Input: part model. Units: mm. Frame: model coordinates. A direction names the side the tool comes from. Give positions to 0.01 mm unless a question says otherwise; leave off trailing zeros. Loops run counter-clockwise (first coordinate to the right, second up) from the corner with the lowest first, then second, coordinate; pieces in that order, holes last.
from build123d import *

# Parameters (mm, degrees)
F0_R          = 25.4
F1_DEPTH      = 19.05
F2_R          = 6.35
F3_DEPTH      = 12.7
F5_DEPTH      = 25.4
F5_DEPTH_BACK = 50.8
F6_W          = 25.4
F6_H          = 25.4
F7_DEPTH      = 25.4
F9_DEPTH      = 115.8426897829


# Not quite as in the source:
# - a pattern or mirror of a feature is missing from the dataset's text; its kind, count and spacing are read off the source's solid


with BuildPart() as f1:
    # F0 (on Top) → F1 (new body)
    with BuildSketch(Plane.XY):
        with BuildLine():
            Line((-35.052, -28.575), (35.052, -28.575))
            Line((35.052, -28.575), (35.052, 28.575))
            ThreePointArc((35.052, 28.575), (28.9292508026, 48.3674518946), (12.7, 61.2453643077))
            Line((12.7, 61.2453643077), (12.7, 79.375))
            Line((12.7, 79.375), (-12.7, 79.375))
            Line((-12.7, 79.375), (-12.7, 61.2453643077))
            ThreePointArc((-12.7, 61.2453643077), (-28.9292508026, 48.3674518946), (-35.052, 28.575))
            Line((-35.052, 28.575), (-35.052, -28.575))
        make_face()
        with Locations((0, 28.575)):
            Circle(F0_R, mode=Mode.SUBTRACT)
    extrude(amount=F1_DEPTH)

    # F2 (on face) → F3 (join)
    with BuildSketch(Plane(origin=(-35.052, 0, 0), x_dir=(0, -1, 0), z_dir=(-1, 0, 0))):
        with BuildLine():
            Line((3.175, 19.05), (28.575, 19.05))
            Line((28.575, 19.05), (28.575, 44.45))
            ThreePointArc((28.575, 44.45), (15.875, 57.15), (3.175, 44.45))
            Line((3.175, 44.45), (3.175, 19.05))
        make_face()
        with Locations((15.875, 44.45)):
            Circle(F2_R, mode=Mode.SUBTRACT)
    f3 = extrude(amount=-F3_DEPTH)

    # F3_copies: F3 across plane
    add(f3.mirror(Plane(origin=(0, 0, 0), x_dir=(0, 0, 1), z_dir=(1, 0, 0))))

    # F4 (on face) → F5 (join, two sides)
    with BuildSketch(Plane(origin=(-12.7, 0, 0), x_dir=(0, -1, 0), z_dir=(-1, 0, 0))) as f5_sk:
        Polygon((-79.375, 0), (-79.375, 19.05), (-178.3617036526, -38.1), (-170.1128116815, -52.3875), align=None)
    extrude(amount=F5_DEPTH)
    extrude(f5_sk.sketch, amount=-F5_DEPTH_BACK)

    # F6 (on face) → F7 (cut)
    with BuildSketch(Plane(origin=(0, 28.092641971, 48.6578832127), x_dir=(1, 0, 0), z_dir=(0, 0.5, 0.8660254038))):
        with Locations((25.4, 71.9157664254)):
            Rectangle(F6_W, F6_H)
        with Locations((-25.4, 71.9157664254)):
            Rectangle(F6_W, F6_H)
        with BuildLine():
            ThreePointArc((-38.1, 135.4157664254), (-26.9407683632, 162.3565347886), (0, 173.5157664254))
            Line((0, 173.5157664254), (-38.1, 173.5157664254))
            Line((-38.1, 173.5157664254), (-38.1, 135.4157664254))
        make_face()
        with BuildLine():
            ThreePointArc((0, 173.5157664254), (26.9407683632, 162.3565347886), (38.1, 135.4157664254))
            Line((38.1, 135.4157664254), (38.1, 173.5157664254))
            Line((38.1, 173.5157664254), (0, 173.5157664254))
        make_face()
    extrude(amount=-F7_DEPTH, mode=Mode.SUBTRACT)

    # F8 (on face) → F9 (cut, through all)
    with BuildSketch(Plane(origin=(0, 28.092641971, 48.6578832127), x_dir=(1, 0, 0), z_dir=(0, 0.5, 0.8660254038))):
        Polygon((21.9970411706, 148.1157664254), (-4.0856e-06, 160.8157664254), (-21.9970493417, 148.1157664254), (-21.9970493417, 122.7157664254), (-4.0856e-06, 110.0157664254), (21.9970411706, 122.7157664254), align=None)
    extrude(amount=-F9_DEPTH, mode=Mode.SUBTRACT)


solid = f1.part
(1) Cut plane B-B (x = 8.5). Return the cut outline in (y, z) (3 decimals), and give its area (3 significant figures).
Values follow:
outline: (-28.575, 0) - (4.639, 0) - (4.639, 19.05) - (-28.575, 19.05) - close; (52.511, 0) - (79.375, 0) - (119.37, -23.091) - (127.619, -8.804) - (79.375, 19.05) - (52.511, 19.05) - close; (154.864, -43.584) - (169.281, -51.907) - (177.53, -37.62) - (163.113, -29.296) - close
area: 2,260 mm2
(2) Cut plane D-D (x = -7). Return the cut outline in (y, z) (3 decimals).
Values follow:
outline: (-28.575, 0) - (4.159, 0) - (4.159, 19.05) - (-28.575, 19.05) - close; (52.991, 0) - (79.375, 0) - (118.62, -22.658) - (126.869, -8.371) - (79.375, 19.05) - (52.991, 19.05) - close; (155.614, -44.017) - (169.551, -52.063) - (177.8, -37.776) - (163.863, -29.729) - close
(3) Ray query, probe 1 along Y at (x, z) = (29, 44) (3 decimals); probe 2 along Z at (x, y) = (-15, -19); probe 3 along Y at (x, z) = (-31.5, 32) (3 decimals). Return the intervals inside material, ascending.
Values follow:
probe 1: y = -28.575 to -22.209, -9.541 to -3.175
probe 2: z = 0 to 19.05
probe 3: y = -28.575 to -3.175
(4) Cut plane A-A (x = -32). Count the separate pieces of the cut face and the enclosed holes in it, and give its area (3 significant figures).
Values follow:
separate pieces: 2
enclosed holes: 1
area: 3,310 mm2
(5) Pin query (flat end, axial travel): pin 1 Ø16.5 at (y, z) = (-15.875, 44.45) entering from -X; pin 2 Ø10 at (x, z) = (-28, -30) entering from -Y; pin 3 Ø20.5 at (y, z) = (-14.5, 44.5) entering from +X. Return the tip coordinate at first contact, or that it passes through.
Values follow:
pin 1: stops at x = -35.05
pin 2: stops at y = 122.68
pin 3: stops at x = 35.05
(6) Cut plane C-C (z = 12). Return the cut outline in (x, y) (3 decimals).
Values follow:
outline: (-35.052, -28.575) - (35.052, -28.575) - (35.052, 28.575) arc R35.052 ccw to (12.7, 61.245) - (12.7, 91.586) - (-12.7, 91.586) - (-12.7, 61.245) arc R35.052 ccw to (-35.052, 28.575) - close; hole circle Ø50.8 at (0, 28.575)
(7) Mould query, pull axis Y, two halves, no side actions, for faces 5 (the flat face through (29, -3.175, 32)), 6 (the flat face through (22.352, -16, 34)), 7 (the cylindrical face through (-28.791, -15.048, 50.746)). Classes: +Y half, -Y half, draft (parallel to the pull), parting line (faces both ways), or undercut.
Values follow:
face 5: +Y half
face 6: draft
face 7: undercut
(8) Reachability of faces 1 (the flat face through (-12.7, 82, 8)), 2 (the flat face through (-35.052, -6, 23)), 3 (the flat face through (21.997, 141, -26)), 4 (the flat face through (35.052, -6, 23)) from +Z, -Z, +X, -X, +Y, -Y: full face, straight path, thin tool, end or side. Return the list, or none.
Values follow:
face 1: +Z, -X
face 2: +Z, -Z, -X, -Y
face 3: none
face 4: +Z, -Z, +X, -Y
